Read the model definition and answer for the solid it produces. Units are mm, in the model's axes. A direction names the side the tool comes from. Coordinates: 2 decimals unless noted, no trailing zeros. Loops run counter-clockwise (first coordinate to the right, second up) from the corner with the lowest first, then second, coordinate; pieces in that order, holes last. Notation, with made-up numbers: (-7.5, 30) -> (46.5, 30) arc R27 cw to (46.5, 60) -> close; hole circle Ø5 at (65.5, -39.5). An arc over 180 degrees is marked (long way). Answer as a JSON object with one key per item and string values. Group by question number.
1) Which of the six approach directions +Z, -Z, +X, -X, +Y, -Y give full straight-line access (tool end or side, diameter ignored) to faces 4 (the face through (-6, 15, 7.099)), 5 (the face through (-3.45, -15.52, 20.46))?
2) Consider probe 1 along Y at (x, z) = (0, 9.25); probe 2 along Y at (x, z) = (1, 17.5); probe 3 along X at (y, z) = (-3, 7.5). Determine where each line is inside the solid, lowest interval first. Write a range as [from, to].
3) Flat-ended cylindrical pins translate along their axes: P1, Ø2, axis at y = 6.5, z = 18, coming from the +X side; P2, Ø10, axis at x = 4, y = 6.5, coming from the +Z side; P3, Ø12, axis at y = 12, z = 20.5, coming from the -X side; P4, Ø3, axis at x = -3.5, z = 7.5, coming from the +Y side. Find the tip coordinate at first contact, or state that the pin passes through.
4) Determine the mould class of faces 1 (the face through (-3.45, -15.52, 2.94)), 2 (the face through (-13.858, -10.626, 11.576)), 3 (the face through (9, -14, 0)) for opening direction Y: released by +Y, released by -Y, zero draft, split by the parting line, or undercut.
5) Section C-C, the plane z = 3.75 is taken. Give the vertices of the cut face in (x, y) (1 decimal), plus the area to 3 significant figures.
from build123d import *

# Parameters (mm, degrees)
SKETCH1_R          = 17.4625
SKETCH1_R_2        = 15.9004
BASE_EXTRUDE_DEPTH = 23.4696
SKETCH2_R          = 16.5735
CUT_EXTRUDE1_DEPTH = 1.524
CUT_EXTRUDE2_START = 1.524
SKETCH3_R          = 16.5735
CUT_EXTRUDE2_DEPTH = 1.524
CHAMFER1_SIZE      = 0.381


with BuildPart() as part:
    # Sketch1 → Base-Extrude (new body)
    with BuildSketch(Plane.XY):
        Circle(SKETCH1_R)
        Circle(SKETCH1_R_2, mode=Mode.SUBTRACT)
    extrude(amount=BASE_EXTRUDE_DEPTH)

    # Sketch2 → Cut-Extrude1 (cut)
    with BuildSketch(Plane.XY.offset(7.0993)):
        Circle(SKETCH2_R)
    extrude(amount=-CUT_EXTRUDE1_DEPTH, mode=Mode.SUBTRACT)

    # Sketch3 → Cut-Extrude2 (cut)
    with BuildSketch(Plane.XY.offset(16.3703).offset(CUT_EXTRUDE2_START)):
        Circle(SKETCH3_R)
    extrude(amount=-CUT_EXTRUDE2_DEPTH, mode=Mode.SUBTRACT)

    # Chamfer1
    chamfer1_edges = [part.edges().sort_by_distance(p)[0] for p in [
        (-17.4625, 0, 0),
        (-17.4625, 0, 23.4696),
        (-15.9004, 0, 0),
        (-15.9004, 0, 23.4696),
    ]]
    chamfer(chamfer1_edges, length=CHAMFER1_SIZE)


solid = part.part
Determined:
{
 "1": {"face 4": "none", "face 5": "+Z, -Z"},
 "2": {"probe 1": "[-17.46, -15.9], [15.9, 17.46]", "probe 2": "[-17.43, -16.54], [16.54, 17.43]", "probe 3": "[-17.2, -15.61], [15.61, 17.2]"},
 "3": {"P1": "x = 16.57", "P2": "through", "P3": "x = -16.4", "P4": "y = 17.35"},
 "4": {"face 1": "undercut", "face 2": "split by the parting line", "face 3": "zero draft"},
 "5": {"outline": "circle Ø34.9 at (0, 0); hole circle Ø31.8 at (0, 0)", "area": "164 mm²"}
}
